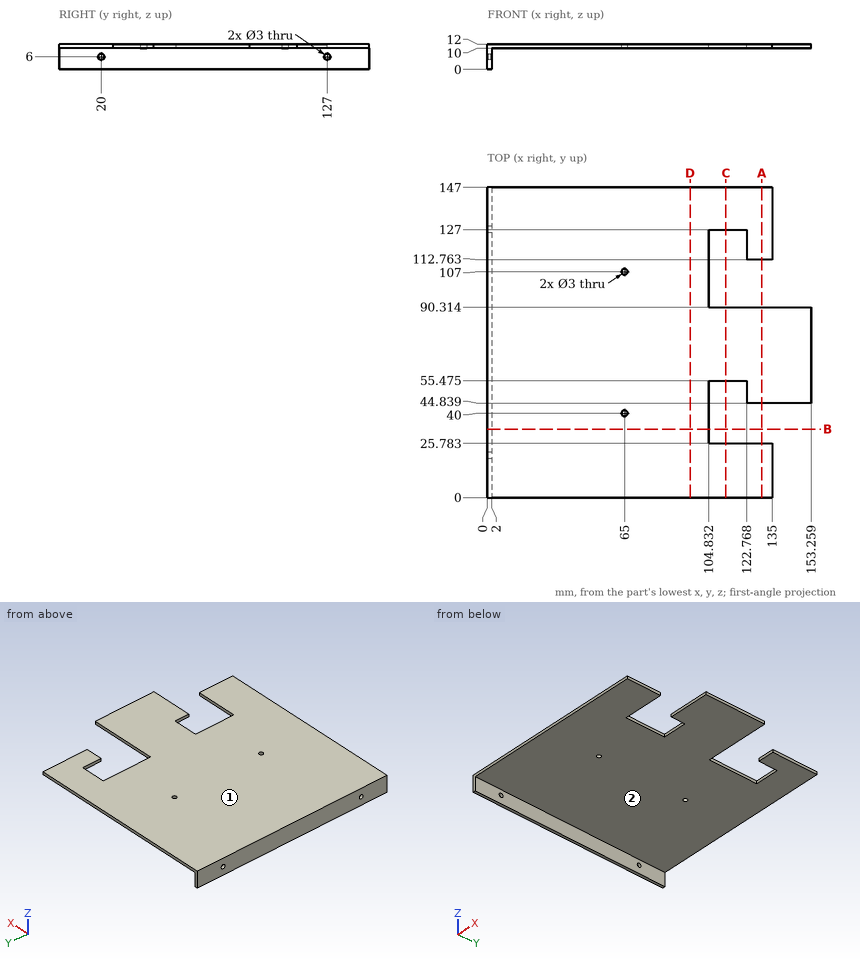
Here's the drawing with two shaded views (mm, measured from the low corner). I have some questions. A direction names the side the tool comes from. Coordinates: 2 decimals unless noted, no trailing zeros. Write each loop counter-clockwise with the first axis right and the second up, starting at its lowest first coordinate (ties: lowest second). Pieces come first, ordered by that corner, then holes. Notation, with made-up numbers: M -15,8.25 L 32,8.25 A16 cw 32,22.25 Z; hole C -8.75,-31 d4. An arc over 180 degrees is marked long. Write item = value, one per line. Start each with the question number.
Q1. If we section it at C-C, the plane x = 113: Write out the boundary of the cut face in (y, z) (1 decimal).
Q2. If we section it at A-A, the plane x = 130: Write out the boundary of the cut face in (y, z), then the cut area to 3 significant figures.
Q3. I'm going to push flat-ended pins straight in: pin 1 (0.6 mm diameter, centred on y = 125, z = 11.5, fed in from +X); pin 2 (3 mm diameter, centred on y = 71.5, z = 5.5, fed in from +X); pin 3 (1 mm diameter, centred on y = 34.5, z = 11, fed in from +X). Where does each tip first touch, or does it pass through?
Q4. If we section it at D-D, the plane x = 96: Write out the boundary of the cut face in (y, z).
Q5. If we section it at B-B, the plane y = 32.5: Write out the boundary of the cut face in (x, z).
Q6. If I drill on L1, parallel to Y at x = 0.6, z = 6; L2, parallel to Z at x = 1.1, y = 20; L3, parallel to Y at x = 65, z = 10.7, over which ranges is the centre line in solid material (lowest first)? Write a range as [from, to].
Q7. On a 3-axis mill with a long thin cutter (end or side, diameter ignored), from which of +Z, -Z, +X, -X, +Y, -Y can I reach the whole of each face in a straight line? I mean the marked faces 1 and 2. Say none if no direction works.
Check sheet entries:
q1.outline = M 0,10 L 25.8,10 L 25.8,12 L 0,12 Z; M 55.5,10 L 90.3,10 L 90.3,12 L 55.5,12 Z; M 127,10 L 147,10 L 147,12 L 127,12 Z
q2.outline = M 0,10 L 25.78,10 L 25.78,12 L 0,12 Z; M 44.84,10 L 90.31,10 L 90.31,12 L 44.84,12 Z; M 112.76,10 L 147,10 L 147,12 L 112.76,12 Z
q2.area = 211 mm²
q3.pin_1 = 135
q3.pin_2 = 2
q3.pin_3 = 104.83
q4.outline = M 0,10 L 147,10 L 147,12 L 0,12 Z
q5.outline = M 0,0 L 2,0 L 2,10 L 104.83,10 L 104.83,12 L 0,12 Z
q6.L1 = [0, 18.5], [21.5, 125.5], [128.5, 147]
q6.L2 = [0, 4.5], [7.5, 12]
q6.L3 = [0, 38.5], [41.5, 105.5], [108.5, 147]
q7.face_1 = +Z, +X, -X, +Y, -Y
q7.face_2 = -Z, +X, +Y, -Y
